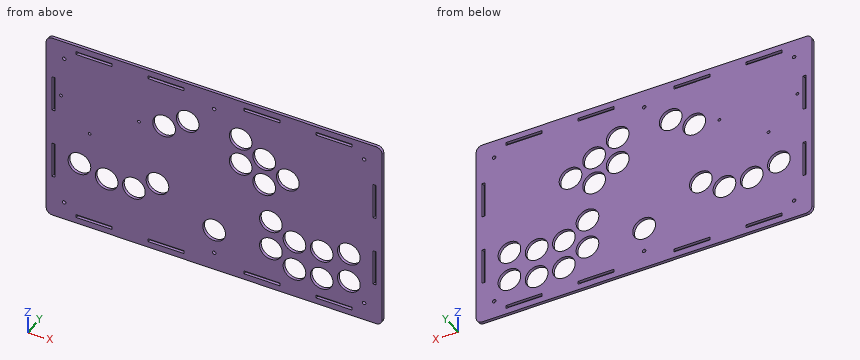
```python
from build123d import *

# Parameters (mm, degrees)
PANEL_PROFILE_2_W        = 355.6
PANEL_PROFILE_2_H        = 203.2
PANEL_PROFILE_DEPTH      = 3.175
RIGHT_HAND_BUTTONS_R     = 12
RIGHT_BUTTONS_DEPTH      = 1
RIGHT_BUTTONS_DEPTH_BACK = 3.175
SKETCH4_R                = 12
C_STICK_DEPTH            = 3.175
START_BUTTON_R           = 12
START_DEPTH              = 3.175
SKETCH7_R                = 12
L_STICK_DEPTH            = 3.175
SKETCH8_R                = 1.8288
CUT_EXTRUDE1_DEPTH       = 10
FILLET1_R                = 6.35
CUT_EXTRUDE2_START       = -4.175
SKETCH9_W                = 38.18
SKETCH9_H                = 3.25
CUT_EXTRUDE2_DEPTH       = 5.175
MIRROR2_START            = -4.175
MIRROR2_COPY_1_SKETCH_W  = 38.18
MIRROR2_COPY_1_SKETCH_H  = 3.25
MIRROR2_COPY_1_DEPTH     = 5.175
CUT_EXTRUDE3_START       = -4.175
SKETCH10_W               = 3.2004
SKETCH10_H               = 38.1254
CUT_EXTRUDE3_DEPTH       = 5.175
MIRROR4_START            = -4.175
MIRROR4_COPY_1_SKETCH_W  = 3.2004
MIRROR4_COPY_1_SKETCH_H  = 38.1254
MIRROR4_COPY_1_DEPTH     = 5.175
SKETCH12_R               = 1.4732
CUT_EXTRUDE4_DEPTH       = 1
CUT_EXTRUDE4_DEPTH_BACK  = 4.175


with BuildPart() as part:
    # Panel Profile 2 → Panel-Profile (new body)
    with BuildSketch(Plane(origin=(0, 0, 0), x_dir=(1, 0, 0), z_dir=(0, 1, 0))):
        Rectangle(PANEL_PROFILE_2_W, PANEL_PROFILE_2_H)
    extrude(amount=-PANEL_PROFILE_DEPTH)

    # Right Hand Buttons → Right Buttons (cut, two sides)
    with BuildSketch(Plane(origin=(0, 0, 0), x_dir=(1, 0, 0), z_dir=(0, 1, 0))) as right_buttons_sk:
        with Locations((60, 56.2)):
            Circle(RIGHT_HAND_BUTTONS_R)
        with Locations((85, 70.6)):
            Circle(RIGHT_HAND_BUTTONS_R)
        with Locations((113.8, 70.6)):
            Circle(RIGHT_HAND_BUTTONS_R)
        with Locations((142.6, 63.4)):
            Circle(RIGHT_HAND_BUTTONS_R)
        with Locations((60, 25)):
            Circle(RIGHT_HAND_BUTTONS_R)
        with Locations((85, 39.4)):
            Circle(RIGHT_HAND_BUTTONS_R)
        with Locations((113.8, 39.4)):
            Circle(RIGHT_HAND_BUTTONS_R)
        with Locations((142.6, 32.2)):
            Circle(RIGHT_HAND_BUTTONS_R)
    extrude(amount=RIGHT_BUTTONS_DEPTH, mode=Mode.SUBTRACT)
    extrude(right_buttons_sk.sketch, amount=-RIGHT_BUTTONS_DEPTH_BACK, mode=Mode.SUBTRACT)

    # Sketch4 → C-Stick (cut)
    with BuildSketch(Plane(origin=(0, 0, 0), x_dir=(1, 0, 0), z_dir=(0, 1, 0))):
        with Locations((53, -43.8)):
            Circle(SKETCH4_R)
        with Locations((53, -15)):
            Circle(SKETCH4_R)
        with Locations((77.941531629, -29.4)):
            Circle(SKETCH4_R)
        with Locations((28.058468371, -29.4)):
            Circle(SKETCH4_R)
        with Locations((28.058468371, -58.2)):
            Circle(SKETCH4_R)
    extrude(amount=-C_STICK_DEPTH, mode=Mode.SUBTRACT)

    # Start Button → Start (cut)
    with BuildSketch(Plane(origin=(0, 0, 0), x_dir=(1, 0, 0), z_dir=(0, 1, 0))):
        with Locations((0, 56.6)):
            Circle(START_BUTTON_R)
    extrude(amount=-START_DEPTH, mode=Mode.SUBTRACT)

    # Sketch7 → L-Stick (cut)
    with BuildSketch(Plane(origin=(0, 0, 0), x_dir=(1, 0, 0), z_dir=(0, 1, 0))):
        with Locations((-142.6, 32.2)):
            Circle(SKETCH7_R)
        with Locations((-113.8, 39.4)):
            Circle(SKETCH7_R)
        with Locations((-85, 39.4)):
            Circle(SKETCH7_R)
        with Locations((-60, 25)):
            Circle(SKETCH7_R)
        with Locations((-53, -43.8)):
            Circle(SKETCH7_R)
        with Locations((-28.058468371, -58.2)):
            Circle(SKETCH7_R)
    extrude(amount=-L_STICK_DEPTH, mode=Mode.SUBTRACT)

    # Sketch8 → Cut-Extrude1 (cut)
    with BuildSketch(Plane(origin=(0, 0, 0), x_dir=(1, 0, 0), z_dir=(0, 1, 0))):
        with Locations((-158.75, 82.55)):
            Circle(SKETCH8_R)
        with Locations((0, 82.55)):
            Circle(SKETCH8_R)
        with Locations((158.75, 82.55)):
            Circle(SKETCH8_R)
        with Locations((-158.75, -82.55)):
            Circle(SKETCH8_R)
        with Locations((0, -82.55)):
            Circle(SKETCH8_R)
        with Locations((158.75, -82.55)):
            Circle(SKETCH8_R)
    extrude(amount=-CUT_EXTRUDE1_DEPTH, mode=Mode.SUBTRACT)

    # Fillet1
    fillet1_edges = [part.edges().sort_by_distance(p)[0] for p in [
        (177.8, -1.5875, 101.6),
        (-177.8, -1.5875, 101.6),
        (-177.8, -1.5875, -101.6),
        (177.8, -1.5875, -101.6),
    ]]
    fillet(fillet1_edges, radius=FILLET1_R)

    # Sketch9 → Cut-Extrude2 (cut)
    with BuildSketch(Plane(origin=(0, 0, 0), x_dir=(1, 0, 0), z_dir=(0, 1, 0)).offset(CUT_EXTRUDE2_START)):
        with Locations((-127, 93.625)):
            Rectangle(SKETCH9_W, SKETCH9_H)
        with Locations((-50.8, 93.625)):
            Rectangle(SKETCH9_W, SKETCH9_H)
    cut_extrude2 = extrude(amount=CUT_EXTRUDE2_DEPTH, mode=Mode.SUBTRACT)

    # Mirror1: Cut-Extrude2 across plane
    add(cut_extrude2.mirror(Plane(origin=(0, 0, 0), x_dir=(0, 0, 1), z_dir=(1, 0, 0))), mode=Mode.SUBTRACT)

    # Mirror2: Cut-Extrude2 across plane
    add(cut_extrude2.mirror(Plane.XY), mode=Mode.SUBTRACT)

    # Mirror2 copy 1 sketch → Mirror2 copy 1 (cut)
    with BuildSketch(Plane(origin=(0, 0, 0), x_dir=(-1, 0, 0), z_dir=(0, 1, 0)).offset(MIRROR2_START)):
        with Locations((-127, 93.625)):
            Rectangle(MIRROR2_COPY_1_SKETCH_W, MIRROR2_COPY_1_SKETCH_H)
        with Locations((-50.8, 93.625)):
            Rectangle(MIRROR2_COPY_1_SKETCH_W, MIRROR2_COPY_1_SKETCH_H)
    extrude(amount=MIRROR2_COPY_1_DEPTH, mode=Mode.SUBTRACT)

    # Sketch10 → Cut-Extrude3 (cut)
    with BuildSketch(Plane(origin=(0, 0, 0), x_dir=(1, 0, 0), z_dir=(0, 1, 0)).offset(CUT_EXTRUDE3_START)):
        with Locations((-169.8498, 38.1)):
            Rectangle(SKETCH10_W, SKETCH10_H)
    cut_extrude3 = extrude(amount=CUT_EXTRUDE3_DEPTH, mode=Mode.SUBTRACT)

    # Mirror3: Cut-Extrude3 across plane
    add(cut_extrude3.mirror(Plane.XY), mode=Mode.SUBTRACT)

    # Mirror4: Cut-Extrude3 across plane
    add(cut_extrude3.mirror(Plane(origin=(0, 0, 0), x_dir=(0, 0, 1), z_dir=(1, 0, 0))), mode=Mode.SUBTRACT)

    # Mirror4 copy 1 sketch → Mirror4 copy 1 (cut)
    with BuildSketch(Plane(origin=(0, 0, 0), x_dir=(-1, 0, 0), z_dir=(0, 1, 0)).offset(MIRROR4_START)):
        with Locations((-169.8498, 38.1)):
            Rectangle(MIRROR4_COPY_1_SKETCH_W, MIRROR4_COPY_1_SKETCH_H)
    extrude(amount=MIRROR4_COPY_1_DEPTH, mode=Mode.SUBTRACT)

    # Sketch12 → Cut-Extrude4 (cut, two sides)
    with BuildSketch(Plane.XZ.offset(3.175)) as cut_extrude4_sk:
        with Locations((-79.6196, 39.06)):
            Circle(SKETCH12_R)
        with Locations((-131.6896, 6.04)):
            Circle(SKETCH12_R)
        with Locations((-162.1696, 39.06)):
            Circle(SKETCH12_R)
    extrude(amount=CUT_EXTRUDE4_DEPTH, mode=Mode.SUBTRACT)
    extrude(cut_extrude4_sk.sketch, amount=-CUT_EXTRUDE4_DEPTH_BACK, mode=Mode.SUBTRACT)


solid = part.part
```
Can you work these out from the model? Positions are in its coordinate system, mm. Round coordinates to 2 decimals unless told otherwise and drop trailing zeros. Loops run counter-clockwise (first coordinate to the right, second up) from the corner with the lowest first, then second, coordinate; pieces in that order, holes last. Notation, with made-up numbers: (-30.75, -20.75) -> (-6.75, -20.75) arc R25 cw to (-6.75, 0.25) -> close; hole circle Ø9 at (-36, 84.25). An arc over 180 degrees is marked (long way). One line per item, written item: value. Start each with the question number.
1. If we section it at C-C, the plane x = -142.6: Write out the boundary of the cut face in (y, z) (3 decimals).
2. If we section it at A-A, the plane x = -85: Write out the boundary of the cut face in (y, z) (3 decimals).
3. If we section it at B-B, the plane x = 53: Write out the boundary of the cut face in (y, z) (3 decimals), then the cut area to 3 significant figures.
4. If we section it at D-D, the plane y = -0.6: Give the number of separate pieces and of enclosed holes in the cut face, then the cut area to 3 significant figures.
5. If I drill on probe 1 along Z at (x, y) = (142, -2.5) (3 decimals); probe 2 along X at (y, z) = (-1.2, 43.8); probe 3 along Z at (x, y) = (-28, -2.7), over which ranges is the centre line in solid material (lowest first)?
6. For pin 1 (14.5 mm diameter, centred on x = 28.06, z = 58.2, fed in from +Y), with a flat end and sliding along its axis, tell me the tip position at first contact or that it passes through.
Calculated:
1. outline: (-3.175, -101.6) -> (0, -101.6) -> (0, -95.25) -> (-3.175, -95.25) -> close; (-3.175, -92) -> (0, -92) -> (0, -44.2) -> (-3.175, -44.2) -> close; (-3.175, -20.2) -> (0, -20.2) -> (0, 92) -> (-3.175, 92) -> close; (-3.175, 95.25) -> (0, 95.25) -> (0, 101.6) -> (-3.175, 101.6) -> close
2. outline: (-3.175, -101.6) -> (0, -101.6) -> (0, -51.4) -> (-3.175, -51.4) -> close; (-3.175, -27.4) -> (0, -27.4) -> (0, 101.6) -> (-3.175, 101.6) -> close
3. outline: (-3.175, -101.6) -> (0, -101.6) -> (0, -95.25) -> (-3.175, -95.25) -> close; (-3.175, -92) -> (0, -92) -> (0, -65.947) -> (-3.175, -65.947) -> close; (-3.175, -46.453) -> (0, -46.453) -> (0, -34.747) -> (-3.175, -34.747) -> close; (-3.175, -15.253) -> (0, -15.253) -> (0, 3) -> (-3.175, 3) -> close; (-3.175, 27) -> (0, 27) -> (0, 31.8) -> (-3.175, 31.8) -> close; (-3.175, 55.8) -> (0, 55.8) -> (0, 92) -> (-3.175, 92) -> close; (-3.175, 95.25) -> (0, 95.25) -> (0, 101.6) -> (-3.175, 101.6) -> close
3. area: 348 mm²
4. separate pieces: 1
4. enclosed holes: 41
4. area: 61,600 mm²
5. probe 1: z = -101.6 to -95.25, -92 to -75.385, -51.415 to -44.185, -20.215 to 92, 95.25 to 101.6
5. probe 2: x = -177.8 to -171.45, -168.25 to -65, -41 to 41, 65 to 168.25, 171.45 to 177.8
5. probe 3: z = -101.6 to 46.2, 70.2 to 101.6
6. pin 1: passes through
